Here's how the part is built. I have some questions about the finished solid (model axes, mm). A direction names the side the tool comes from. Give positions to 0.01 mm unless a question says otherwise; leave off trailing zeros. Loops run counter-clockwise (first coordinate to the right, second up) from the corner with the lowest first, then second, coordinate; pieces in that order, holes last.
Q1. If we section it at A-A (y = 5.25): Please give me the cut outline in (x, z), plus the area to 3 significant figures.
Q2. We'd pull the mould along X, two halves only. Please class faces 1 (the face through (-4.219, -3.375, 6.261)), 2 (the face through (-1.964, 5.005, 6.261)), 3 (the face through (5.317, -0.802, 6.261)): +X half, -X half, draft (parallel to the pull), parting line (faces both ways), or undercut.
Q3. I need wall thicknesses on line 1 (X direction, y = -4.5, z = 10.25); line 2 (Y direction, x = 3.75, z = 9.75); line 3 (Y direction, x = 5, z = 1). Which ranges of each line are inside material? Lowest first, please.
Q4. If we section it at B-B (x = 5): Please give me the cut outline in (y, z), plus the area to 3 significant figures.
Q5. Will these pins go through, and if not, where does the flat tip stop? P1, Ø5, axis at x = -4, z = 8.5, coming from the +Y side; P2, Ø1, axis at y = 2.5, z = 3.5, coming from the -X side; P3, Ø2, axis at y = -4, z = 2.5, coming from the +X side.
Q6. For faces 4 (the face through (-6.13, -1.65, 6.26)), 5 (the face through (-3.375, 4.219, 6.261)), 6 (the face through (-4.2, 3.35, 6.26)), 7 (the face through (0.813, -5.342, 6.261)), 8 (the face through (1.964, -5.005, 6.261)), which set-ups out of +Z, -Z, +X, -X, +Y, -Y let a thin tool reach every point of the face, with its end or its side?
from build123d import *

# Parameters (mm, degrees)
F0_R     = 6.35
F0_R_2   = 3.175
F1_DEPTH = 12.7
F2_R     = 6.699885
F3_DEPTH = 12.7


with BuildPart() as f1:
    # F0 (on Top) → F1 (new body)
    with BuildSketch(Plane.XY):
        Circle(F0_R)
        Circle(F0_R_2, mode=Mode.SUBTRACT)
    extrude(amount=F1_DEPTH)

    # F2 (on Top) → F3 (cut, through all)
    with BuildSketch(Plane.XY):
        Circle(F2_R)
        with BuildLine():
            ThreePointArc((-4.428085, -0.387407), (-4.440769, -0.193888), (-4.445, 0))
            ThreePointArc((-4.445, 0), (-4.440769, 0.193888), (-4.428085, 0.387407))
            Line((-4.428085, 0.387407), (-6.230181, 1.227738))
            ThreePointArc((-6.230181, 1.227738), (-6.133629, 1.643501), (-6.009364, 2.051838))
            Line((-6.009364, 2.051838), (-4.028538, 1.878538))
            ThreePointArc((-4.028538, 1.878538), (-3.942763, 2.052473), (-3.849483, 2.2225))
            ThreePointArc((-3.849483, 2.2225), (-3.748875, 2.388297), (-3.641131, 2.549547))
            Line((-3.641131, 2.549547), (-4.781626, 4.178343))
            ThreePointArc((-4.781626, 4.178343), (-4.490128, 4.490128), (-4.178343, 4.781626))
            Line((-4.178343, 4.781626), (-2.549547, 3.641131))
            ThreePointArc((-2.549547, 3.641131), (-2.388297, 3.748875), (-2.2225, 3.849483))
            ThreePointArc((-2.2225, 3.849483), (-2.052473, 3.942763), (-1.878538, 4.028538))
            Line((-1.878538, 4.028538), (-2.051838, 6.009364))
            ThreePointArc((-2.051838, 6.009364), (-1.643501, 6.133629), (-1.227738, 6.230181))
            Line((-1.227738, 6.230181), (-0.387407, 4.428085))
            ThreePointArc((-0.387407, 4.428085), (-0.193888, 4.440769), (0, 4.445))
            ThreePointArc((0, 4.445), (0.193888, 4.440769), (0.387407, 4.428085))
            Line((0.387407, 4.428085), (1.227738, 6.230181))
            ThreePointArc((1.227738, 6.230181), (1.643501, 6.133629), (2.051838, 6.009364))
            Line((2.051838, 6.009364), (1.878538, 4.028538))
            ThreePointArc((1.878538, 4.028538), (2.052473, 3.942763), (2.2225, 3.849483))
            ThreePointArc((2.2225, 3.849483), (2.388297, 3.748875), (2.549547, 3.641131))
            Line((2.549547, 3.641131), (4.178343, 4.781626))
            ThreePointArc((4.178343, 4.781626), (4.490128, 4.490128), (4.781626, 4.178343))
            Line((4.781626, 4.178343), (3.641131, 2.549547))
            ThreePointArc((3.641131, 2.549547), (3.748875, 2.388297), (3.849483, 2.2225))
            ThreePointArc((3.849483, 2.2225), (3.942763, 2.052473), (4.028538, 1.878538))
            Line((4.028538, 1.878538), (6.009364, 2.051838))
            ThreePointArc((6.009364, 2.051838), (6.133629, 1.643501), (6.230181, 1.227738))
            Line((6.230181, 1.227738), (4.428085, 0.387407))
            ThreePointArc((4.428085, 0.387407), (4.440769, 0.193888), (4.445, 0))
            ThreePointArc((4.445, 0), (4.440769, -0.193888), (4.428085, -0.387407))
            Line((4.428085, -0.387407), (6.230181, -1.227738))
            ThreePointArc((6.230181, -1.227738), (6.133629, -1.643501), (6.009364, -2.051838))
            Line((6.009364, -2.051838), (4.028538, -1.878538))
            ThreePointArc((4.028538, -1.878538), (3.942763, -2.052473), (3.849483, -2.2225))
            ThreePointArc((3.849483, -2.2225), (3.748875, -2.388297), (3.641131, -2.549547))
            Line((3.641131, -2.549547), (4.781626, -4.178343))
            ThreePointArc((4.781626, -4.178343), (4.490128, -4.490128), (4.178343, -4.781626))
            Line((4.178343, -4.781626), (2.549547, -3.641131))
            ThreePointArc((2.549547, -3.641131), (2.388297, -3.748875), (2.2225, -3.849483))
            ThreePointArc((2.2225, -3.849483), (2.052473, -3.942763), (1.878538, -4.028538))
            Line((1.878538, -4.028538), (2.051838, -6.009364))
            ThreePointArc((2.051838, -6.009364), (1.643501, -6.133629), (1.227738, -6.230181))
            Line((1.227738, -6.230181), (0.387407, -4.428085))
            ThreePointArc((0.387407, -4.428085), (0.193888, -4.440769), (0, -4.445))
            ThreePointArc((0, -4.445), (-0.193888, -4.440769), (-0.387407, -4.428085))
            Line((-0.387407, -4.428085), (-1.227738, -6.230181))
            ThreePointArc((-1.227738, -6.230181), (-1.643501, -6.133629), (-2.051838, -6.009364))
            Line((-2.051838, -6.009364), (-1.878538, -4.028538))
            ThreePointArc((-1.878538, -4.028538), (-2.052473, -3.942763), (-2.2225, -3.849483))
            ThreePointArc((-2.2225, -3.849483), (-2.388297, -3.748875), (-2.549547, -3.641131))
            Line((-2.549547, -3.641131), (-4.178343, -4.781626))
            ThreePointArc((-4.178343, -4.781626), (-4.490128, -4.490128), (-4.781626, -4.178343))
            Line((-4.781626, -4.178343), (-3.641131, -2.549547))
            ThreePointArc((-3.641131, -2.549547), (-3.748875, -2.388297), (-3.849483, -2.2225))
            ThreePointArc((-3.849483, -2.2225), (-3.942763, -2.052473), (-4.028538, -1.878538))
            Line((-4.028538, -1.878538), (-6.009364, -2.051838))
            ThreePointArc((-6.009364, -2.051838), (-6.133629, -1.643501), (-6.230181, -1.227738))
            Line((-6.230181, -1.227738), (-4.428085, -0.387407))
        make_face(mode=Mode.SUBTRACT)
    extrude(amount=F3_DEPTH, mode=Mode.SUBTRACT)


solid = f1.part
Check sheet entries:
1. outline: (-1.99, 0) - (-0.77, 0) - (-0.77, 12.7) - (-1.99, 12.7) - close; (0.77, 0) - (1.99, 0) - (1.99, 12.7) - (0.77, 12.7) - close
1. area: 30.9 mm2
2. face 1: -X half
2. face 2: undercut
2. face 3: +X half
3. line 1: x = -4.48 to -3.78, -1.92 to -0.42, 0.42 to 1.92, 3.78 to 4.48
3. line 2: y = -4.48 to -2.71, -2.39 to 2.39, 2.71 to 4.48
3. line 3: y = -1.96 to -0.65, 0.65 to 1.96
4. outline: (-1.96, 0) - (-0.65, 0) - (-0.65, 12.7) - (-1.96, 12.7) - close; (0.65, 0) - (1.96, 0) - (1.96, 12.7) - (0.65, 12.7) - close
4. area: 33.3 mm2
5. P1: stops at y = 6.17
5. P2: stops at x = -6.03
5. P3: stops at x = 4.78
6. face 4: +Z, -Z, -X, -Y
6. face 5: +Z, -Z, +Y
6. face 6: +Z, -Z, -X
6. face 7: +Z, -Z, -Y
6. face 8: +Z, -Z
